Model file for the job. Use its own axes, mm. A direction names the side the tool comes from. Round coordinates to 2 decimals unless told otherwise and drop trailing zeros. Order: outer loops, then holes, each group sorted by start corner. A loop starts at its lowest first (then second) coordinate and runs counter-clockwise, first axis right, second up. Notation, with made-up numbers: M -29.5,71.5 L 0.5,71.5 A23 ccw 0.5,103.5 Z; hole C 49,41.25 d8. An arc over 180 degrees is marked long. Return JSON: item names as keys, results as strings. Group by question number.
Item 1: Which spindle directions (+Z, -Z, +X, -X, +Y, -Y) get a long thin tool onto all of the face, cutting with end or side? Do faces 1 (the face through (-8, 18, 7.301)), 2 (the face through (-8, 60, 7.301)), 3 (the face through (-41, 39, 83.501)). Say none if no direction does.
Item 2: Slice it at A-A on x = -13. Write the cut outline in (y, z), then the cut area to 3 significant figures.
Item 3: Probe line 1 along Z through (x, y) = (-35.5, 63); line 2 along X through (y, z) = (7, 15.5); line 3 along Y through (x, z) = (-25.5, 26.5). List the from-to ranges inside material, lowest first.
Item 4: Slice it at C-C on y = 56.5. Write the cut outline in (x, z).
Item 5: Pin check, flat tips, straight feed: pin 1 Ø9.5 at (x, y) = (-6.5, 61.5) entering from +Z; pin 2 Ø3 at (y, z) = (22.5, 14.5) entering from +X; pin 3 Ø5 at (x, z) = (-13, 22.5) entering from -Y. Stop position of each tip, or through.
Item 6: Slice it at B-B on z = 47. Write the cut outline in (x, y), then the cut area to 3 significant figures.
from build123d import *

# Parameters (mm, degrees)
F0_W     = 67.6434636116
F0_H     = 7.3007261381
F1_DEPTH = 76.2
F2_W     = 9.6846371889
F2_H     = 76.2
F3_DEPTH = 76.2
F4_W     = 57.9588264227
F4_H     = 8.5687600076
F5_DEPTH = 76.2
F7_DEPTH = 40.2453660319


with BuildPart() as f1:
    # F0 (on Front) → F1 (new body)
    with BuildSketch(Plane.XZ):
        with Locations((-12.3665370047, 3.650363069)):
            Rectangle(F0_W, F0_H)
    extrude(amount=-F1_DEPTH)

    # F2 (on face) → F3 (join)
    with BuildSketch(Plane.XY.offset(7.3007261381)):
        with Locations((-41.3459502161, 38.1)):
            Rectangle(F2_W, F2_H)
    extrude(amount=F3_DEPTH)

    # F4 (on face) → F5 (join)
    with BuildSketch(Plane.XY.offset(7.3007261381)):
        with Locations((-7.5242184103, 40.2400139719)):
            Rectangle(F4_W, F4_H)
    extrude(amount=F5_DEPTH)

    # F6 (on face) → F7 (cut, through all)
    with BuildSketch(Plane.XZ.offset(-35.9556339681)):
        Polygon((21.4551948011, 83.5007261381), (-36.5036316216, 83.5007261381), (21.4551948011, 7.3007261381), align=None)
    extrude(amount=-F7_DEPTH, mode=Mode.SUBTRACT)


solid = f1.part
Output values:
{
 "1": {"face 1": "+Z, +X, -Y", "face 2": "+Z, +X, +Y", "face 3": "+Z, +X, -X, +Y, -Y"},
 "2": {"outline": "M 0,0 L 76.2,0 L 76.2,7.3 L 44.52,7.3 L 44.52,52.6 L 35.96,52.6 L 35.96,7.3 L 0,7.3 Z", "area": "944 mm²"},
 "3": {"line 1": "0 to 7.3", "line 2": "-46.19 to -36.5", "line 3": "35.96 to 44.52"},
 "4": {"outline": "M -46.19,0 L 21.46,0 L 21.46,7.3 L -36.5,7.3 L -36.5,83.5 L -46.19,83.5 Z"},
 "5": {"pin 1": "z = 7.3", "pin 2": "x = -36.5", "pin 3": "y = 35.96"},
 "6": {"outline": "M -46.19,0 L -36.5,0 L -36.5,35.96 L -8.74,35.96 L -8.74,44.52 L -36.5,44.52 L -36.5,76.2 L -46.19,76.2 Z", "area": "976 mm²"}
}
